Could you check a few things on this drawing? It's one solid part, dimensions in mm from its lowest x, y, z. Give positions to 0.01 mm unless a question says otherwise; leave off trailing zeros. Loops run counter-clockwise (first coordinate to the right, second up) from the corner with the lowest first, then second, coordinate; pieces in that order, holes last. Notation, with made-up numbers: M 58.25,-4.5 L 96.25,-4.5 A20 cw 96.25,1.5 Z; hole C 33.25,66.25 d6. An arc over 180 degrees is marked long. Answer as CSV lines item,"result". Start each with the question number.
Item 1: I want a section at A-A on z = 3. List the corners of the cut face in (x, y) for me (1 decimal).
Item 2: If I drill on line 1 along X through (y, z) = (0.65, 2); line 2 along X through (y, z) = (2.3, 30); line 3 along Z through (x, y) = (67.5, 1.15) (1 decimal), over which ranges is the centre line in solid material (lowest first)? Write a range as from..to.
Item 3: Will this pin go through, and if not, where does the flat tip stop? P1, Ø1.3, axis at y = 1.5, z = 30, coming from the -X side.
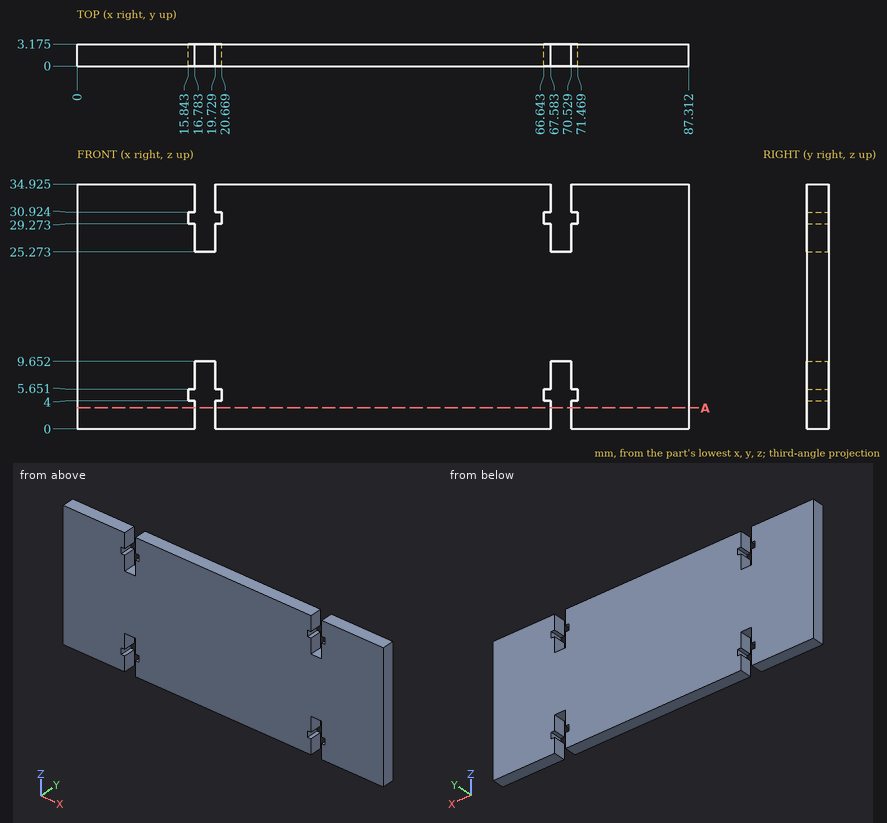
Result:
1,outline,"M 0,0 L 16.8,0 L 16.8,3.2 L 0,3.2 Z; M 19.7,0 L 67.6,0 L 67.6,3.2 L 19.7,3.2 Z; M 70.5,0 L 87.3,0 L 87.3,3.2 L 70.5,3.2 Z"
2,line 1,"0..16.78, 19.73..67.58, 70.53..87.31"
2,line 2,"0..15.84, 20.67..66.64, 71.47..87.31"
2,line 3,"0..4, 5.7..29.3, 30.9..34.9"
3,P1,"x = 0"
